Design review of the part built by this model. Coordinates are the model's own, in mm. A direction names the side the tool comes from. Give positions to 0.01 mm unless a question says otherwise; leave off trailing zeros. Order: outer loops, then holes, each group sorted by start corner. A loop starts at its lowest first (then second) coordinate and runs counter-clockwise, first axis right, second up. Notation, with made-up numbers: (-10, 45.5) -> (43, 45.5) arc R17 cw to (43, 72.5) -> close; hole circle Ø8 at (4.5, 38). An arc over 180 degrees is marked (long way). Use a Markdown table: item, result. Add a question column.
```python
from build123d import *

# Parameters (mm, degrees)
SKETCH1_W           = 19.05
SKETCH1_H           = 19.05
BOSS_EXTRUDE2_DEPTH = 6.35
SKETCH8_W           = 217.17
SKETCH8_H           = 38.1
BOSS_EXTRUDE4_DEPTH = 6.35
SKETCH8_5_W         = 217.17
SKETCH8_5_H         = 38.1
BOSS_EXTRUDE5_DEPTH = 6.4262
SKETCH9_W           = 19.05
SKETCH9_H           = 38.1
LPATTERN3_COUNT     = 11
LPATTERN3_PITCH     = 19.812
SKETCH15_R          = 12.192
BOSS_EXTRUDE6_DEPTH = 6.35


with BuildPart() as part:
    # Sketch1 → Boss-Extrude2 (new body)
    with BuildSketch(Plane(origin=(0, 0, 0), x_dir=(1, 0, 0), z_dir=(0, 1, 0))):
        with Locations((9.525, -9.525)):
            Rectangle(SKETCH1_W, SKETCH1_H)
    extrude(amount=BOSS_EXTRUDE2_DEPTH)

    # Sketch8 → Boss-Extrude4 (add)
    with BuildSketch(Plane(origin=(0, 0, 0), x_dir=(1, 0, 0), z_dir=(0, 1, 0))):
        with Locations((108.585, -9.525)):
            Rectangle(SKETCH8_W, SKETCH8_H)
    extrude(amount=BOSS_EXTRUDE4_DEPTH)

    # Sketch8_5 → Boss-Extrude5 (add)
    with BuildSketch(Plane(origin=(0, 0, 0), x_dir=(1, 0, 0), z_dir=(0, 1, 0))):
        with Locations((108.585, -9.525)):
            Rectangle(SKETCH8_5_W, SKETCH8_5_H)
    extrude(amount=-BOSS_EXTRUDE5_DEPTH)

    # Sketch9 → Loft3 section 0
    with BuildSketch(Plane(origin=(0, 6.35, 0), x_dir=(1, 0, 0), z_dir=(0, 1, 0)), mode=Mode.PRIVATE) as loft3_s0:
        with Locations((9.525, -9.525)):
            Rectangle(SKETCH9_W, SKETCH9_H)
    loft3 = loft([loft3_s0.sketch, Vertex(9.525, 26.0731, 19.05)])

    # LPattern3: Loft3 ×11
    with Locations(*[(i * LPATTERN3_PITCH, 0, 0) for i in range(1, LPATTERN3_COUNT)]):
        add(loft3)

    # Sketch15 → Boss-Extrude6 (add)
    with BuildSketch(Plane.XZ.offset(6.4262)):
        with Locations((179.07, 9.525)):
            Circle(SKETCH15_R)
        with Locations((38.1, 9.525)):
            Circle(SKETCH15_R)
        with Locations((108.585, 9.525)):
            Circle(SKETCH15_R)
    extrude(amount=BOSS_EXTRUDE6_DEPTH)


solid = part.part
```
1) Add section A-A (y = -8.5). Give the boundary of the cut face in (x, z) (3 decimals), then the cut area to 3 significant figures.
2) Machinability: for faces 4 (the cylindrical face through (120.214, -9.557, 13.187)), 5 (the flat face through (148.076, 14.158, 24.804)), 6 (the flat face through (155.02, 11.97, 14.03)), which of the approach directions +Z, -Z, +X, -X, +Y, -Y give a long, thin tool a straight path to every point of the face, cutting with its end or side? Answer none if there is none.
3) Insertion check: pin 1 (12 mm diameter, centred on x = 26, z = -4.5, fed in from -Y); pin 2 (1.5 mm diameter, centred on x = 117, z = 22.5, fed in from +Y); pin 3 (0.8 mm diameter, centred on x = 178, z = 0, fed in from +Y); pin 4 (4 mm diameter, centred on y = 13, z = -4.5, fed in from -X). Each pin has a flat end and moves straight along its axis. Give the tip position at first contact, or say it passes through.
4) For L1, parallel to Y at x = 66.5, z = 18.5; L2, parallel to Y at x = 170, z = 18.5; L3, parallel to Z at x = 48, y = 12, list the stretches that pass through material, from the lowest coordinate up. Write a range as [from, to].
5) The part is to be moulded in two halves that separate along X. For faces 1 (the flat face through (42.34, 11.97, 13.49)), 2 (the flat face through (187.97, 14.16, 1.79)), 3 (the flat face through (214.457, 11.967, 14.025)), say which applies: +X half, -X half, draft (parallel to the pull), parting line (faces both ways), or undercut.
Worked answers:
| question | item | result |
|---|---|---|
| 1 | outline | circle Ø24.384 at (38.1, 9.525); circle Ø24.384 at (108.585, 9.525); circle Ø24.384 at (179.07, 9.525) |
| 1 | area | 1,400 mm^2 |
| 2 | face 4 | -Y |
| 2 | face 5 | +Z, +X, -X, +Y |
| 2 | face 6 | +Z, -Z, +Y |
| 3 | pin 1 | y = -6.43 |
| 3 | pin 2 | y = 10.2 |
| 3 | pin 3 | y = 6.54 |
| 3 | pin 4 | through |
| 4 | L1 | [-6.43, 20.98] |
| 4 | L2 | [-6.43, 21.98] |
| 4 | L3 | [-1.34, 25.85] |
| 5 | face 1 | undercut |
| 5 | face 2 | draft |
| 5 | face 3 | +X half |
